Input: part model. Units: mm. Frame: model coordinates. Give positions to 0.01 mm unless a question says otherwise; leave off trailing zeros. Loops run counter-clockwise (first coordinate to the right, second up) from the corner with the lowest first, then second, coordinate; pieces in that order, holes last.
from build123d import *

# Parameters (mm, degrees)
F0_R     = 5
F1_DEPTH = 8


with BuildPart() as f1:
    # F0 (on Front) → F1 (new body)
    with BuildSketch(Plane.XZ):
        Polygon((8.5, -4.907477), (8.5, 4.907477), (0, 9.814955), (-8.5, 4.907477), (-8.5, -4.907477), (0, -9.814955), align=None)
        Circle(F0_R, mode=Mode.SUBTRACT)
    extrude(amount=F1_DEPTH)

    # F2 (on Top) → F3 (revolve, cut)
    with BuildSketch(Plane.XY):
        Polygon((11.583601, -1.780318), (11.583601, 0), (8.5, 0), align=None)
        Polygon((11.583601, -6.219682), (8.5, -8), (11.583601, -8), align=None)
    revolve(axis=Axis((0, -4, 0), (0, -1, 0)), mode=Mode.SUBTRACT)


solid = f1.part
(1) Mould query, pull axis Z, two halves, no side actions, for faces 1 (the cylindrical face through (-1.08, -3.94, -4.88)), 2 (the conical face through (7.649, -0.185, 4.391)), 3 (the conical face through (-7.649, -0.185, -4.391)). Classes: +Z half, -Z half, draft (parallel to the pull), parting line (faces both ways), or undercut.
Values follow:
face 1: undercut
face 2: +Z half
face 3: -Z half
(2) Ray query, probe 1 along X at (y, z) = (-1.5, -0.5); probe 2 along X at (y, z) = (-3.75, -2.5); probe 3 along Z at (x, y) = (-0.5, -0.5). Return the intervals inside material, ascending.
Values follow:
probe 1: x = -8.5 to -4.97, 4.97 to 8.5
probe 2: x = -8.5 to -4.33, 4.33 to 8.5
probe 3: z = -9.35 to -4.97, 4.97 to 9.35
(3) Cut plane A-A (y = -6). Return the cut outline in (x, z), and give its area (3 significant figures).
Values follow:
outline: (-8.5, -4.91) - (0, -9.81) - (8.5, -4.91) - (8.5, 4.91) - (0, 9.81) - (-8.5, 4.91) - close; hole circle Ø10 at (0, 0)
area: 172 mm2
